Geometry check sheet. Reference: the model listing, model coordinates, mm. Face numbers are marked on the shaded views. A direction names the side the tool comes from. Coordinates: 2 decimals unless noted, no trailing zeros. Loops run counter-clockwise (first coordinate to the right, second up) from the corner with the lowest first, then second, coordinate; pieces in that order, holes last. Notation, with made-up numbers: (-29.75, -26.75) - (11.25, -26.75) arc R31 ccw to (11.25, 8.25) - close; hole circle Ø8 at (23, 89). An arc over 180 degrees is marked (long way). Write item = value, one per line. Start each with the question number.
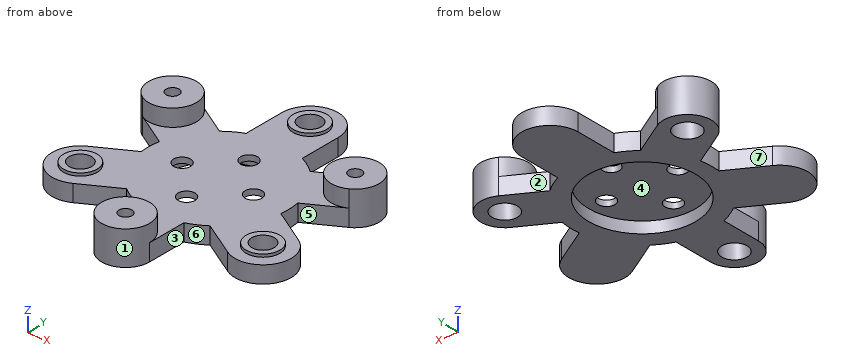
Autodesk Inventor part; units mm, degrees
ref_plane "YZ Plane" through (0, 0, 0) normal (1, 0, 0) x (0, 1, 0)
ref_plane "XZ Plane" through (0, 0, 0) normal (0, 1, 0) x (-1, 0, 0)
ref_plane "XY Plane" through (0, 0, 0) normal (0, 0, 1) x (1, 0, 0)
sketch "Skizze1" plane through (0, 0, 0) normal (0, 0, 1) x (1, 0, 0)
  circle A0 centre (0, 0) radius 18.75 construction
  circle A1 centre (0, 0) radius 9.5
  circle A2 centre (0, 18.75) radius 2
  line L0 (0, 0) -> (-16.238, -9.375) construction
  line L1 (0, 33.1) -> (0, -32.35) construction
  line L2 (-32.2953, 0) -> (32.2953, 0) construction
  circle A3 centre (0, 0) radius 6.35 construction
  circle A4 centre (0, 6.35) radius 1.5
  circle A5 centre (0, -6.35) radius 1.5
  circle A6 centre (6.35, 0) radius 1.5
  circle A7 centre (-6.35, 0) radius 1.5
  arc A8 (-5, 11.4564) -> (5, 11.4564) centre (0, 0) ccw
  arc A9 (5, 18.75) -> (-5, 18.75) centre (0, 18.75) ccw
  line L3 (-5, 18.75) -> (-5, 11.4564)
  line L4 (5, 18.75) -> (5, 11.4564)
  circle A10 centre (16.238, -9.375) radius 2
  arc A11 (13.738, -13.7051) -> (18.738, -5.0449) centre (16.238, -9.375) ccw
  line L5 (18.738, -5.0449) -> (12.4216, -1.3981)
  line L6 (13.738, -13.7051) -> (7.4216, -10.0583)
  circle A12 centre (-16.238, -9.375) radius 2
  arc A13 (-18.738, -5.0449) -> (-13.738, -13.7051) centre (-16.238, -9.375) ccw
  line L7 (-18.738, -5.0449) -> (-12.4216, -1.3981)
  line L8 (-13.738, -13.7051) -> (-7.4216, -10.0583)
  circle A14 centre (0, 18.75) radius 3
  circle A15 centre (16.238, -9.375) radius 3
  circle A16 centre (-16.238, -9.375) radius 3
  circle A17 centre (0, -18.75) radius 1.15
  circle A18 centre (16.238, 9.375) radius 1.15
  circle A19 centre (-16.238, 9.375) radius 1.15
  circle A20 centre (16.238, 9.375) radius 2.25
  circle A21 centre (0, -18.75) radius 2.25
  circle A22 centre (-16.238, 9.375) radius 2.25
  arc A23 (18.363, 5.6944) -> (14.113, 13.0556) centre (16.238, 9.375) ccw
  arc A24 (-4.25, -18.75) -> (4.25, -18.75) centre (0, -18.75) ccw
  arc A25 (-14.113, 13.0556) -> (-18.363, 5.6944) centre (-16.238, 9.375) ccw
  line L9 (18.363, 5.6944) -> (12.3054, 2.1971)
  line L10 (14.113, 13.0556) -> (8.0554, 9.5583)
  line L11 (4.25, -11.7553) -> (4.25, -18.75)
  line L12 (-4.25, -11.7553) -> (-4.25, -18.75)
  line L13 (-8.0554, 9.5583) -> (-14.113, 13.0556)
  line L14 (-12.3054, 2.1971) -> (-18.363, 5.6944)
  circle A26 centre (0, -18.75) radius 4.25
  circle A27 centre (16.238, 9.375) radius 4.25
  circle A28 centre (-16.238, 9.375) radius 4.25
  dimension "d0" = 37.5
  dimension "d1" = 4
  dimension "d2" = 30
  dimension "d3" = 19
  dimension "d4" = 12.7
  dimension "d5" = 3
  dimension "d7" = 3
  dimension "d8" = 3
  dimension "d17" = 1
  dimension "d20" = 2.3
  dimension "d22" = 2
  dimension "d23" = 4.5
extrude "Extrusion1" add sketch "Skizze1" along normal blind 3 contours A1 | A2 | L3 A9 L4 A8 | A8 L14 A28 L13 | A28 A25 | A8 L8 A13 L7 | L10 A27 L9 A8 | A8 L11 A26 L12 | A23 A27 | A26 A24 | L5 A11 L6 A8 | A10 | A12 | A14 | A15 | A16
extrude "Extrusion3" cut sketch "Skizze1" along normal blind 2 contours A1
extrude "Extrusion4" cut sketch "Skizze1" against normal blind 2 from surface at 3 contours A2 | A10 | A12
extrude "Extrusion5" add sketch "Skizze1" along normal blind 0.5 from surface at 3 contours A14 | A15 | A16
extrude "Extrusion6" add sketch "Skizze1" along normal blind 3 from surface at 3 contours A28 A25 | A23 A27 | A26 A24 | A20 | A21 | A22
properties part number "PlanetaryHolderTop"
(1) Draft check along X on the marked faces 5, 6 and 7. Enter one of: pulls with the +X half, pulls with the -X half, needs draft (parallel to the pull), parting line crosses it, or undercut.
(2) Depth check by flat-ended pin: pin 1 (3.5 mm diameter, centred on x = 0, y = -18.75, fed in from -Z); pin 2 (6.5 mm diameter, centred on x = -1, y = 20, fed in from +Z); pin 3 (3 mm diameter, centred on y = 7.5, z = 2.5, fed in from +X). Enter the tip coordinate at first touch or a pass-through.
(3) Sectioned sample at B-B on z = 5.35. Enter the section's corners in (x, y) (3 decimals), plus the area to 3 significant figures.
(4) Scan lines: line 1 (Y direction, x = 0, z = 2.7); line 2 (Z direction, x = 3.5, y = 7); line 3 (Y direction, x = 17.5, z = 2.7). Record each from-to range of solid material in increasing order.
(5) Sectioned sample at C-C on x = 0. Count the separate pieces of the cut face and the enclosed holes in it, plus the area to 4 significant figures.
(6) Tool access check on the marked faces 1, 2, 3 and 4. Record the directions out of +Z, -Z, +X, -X, +Y, -Y that give a thin tool (end or side, any length) a straight path to the whole face; none if there is none.
(7) Sectioned sample at A-A on y = 0. Enter the section's corners in (x, z).
(8) Sectioned sample at D-D on x = 6.35. Enter the section's corners in (y, z).
Working result:
q1.face_5 = pulls with the +X half
q1.face_6 = undercut
q1.face_7 = pulls with the -X half
q2.pin_1 = 3
q2.pin_2 = 3.5
q2.pin_3 = 20.47
q3.outline = (-18.363, 5.694) arc R4.25 ccw to (-14.113, 13.056) arc R4.25 ccw to start; circle Ø8.5 at (0, -18.75); circle Ø8.5 at (16.238, 9.375); hole circle Ø2.3 at (-16.238, 9.375); hole circle Ø2.3 at (0, -18.75); hole circle Ø2.3 at (16.238, 9.375)
q3.area = 158 mm2
q4.line_1 = -23 to -21, -16.5 to -7.85, -4.85 to 4.85, 7.85 to 16.75, 20.75 to 23.75
q4.line_2 = 2 to 3
q4.line_3 = -14.21 to -10.93, -7.82 to -4.33, 5.2 to 7.51, 11.24 to 13.43
q5.separate_pieces = 4
q5.enclosed_holes = 0
q5.area = 94.35 mm2
q6.face_1 = +Z
q6.face_2 = +Z, -Z, +Y
q6.face_3 = +Z, -Z, -Y
q6.face_4 = -Z
q7.outline = (-12.5, 0) - (-9.5, 0) - (-9.5, 2) - (-7.85, 2) - (-7.85, 3) - (-12.5, 3) - close; (-4.85, 2) - (4.85, 2) - (4.85, 3) - (-4.85, 3) - close; (7.85, 2) - (9.5, 2) - (9.5, 0) - (12.5, 0) - (12.5, 3) - (7.85, 3) - close
q8.outline = (-10.77, 0) - (-7.07, 0) - (-7.07, 2) - (-1.5, 2) - (-1.5, 3) - (-10.77, 3) - close; (1.5, 2) - (7.07, 2) - (7.07, 0) - (10.77, 0) - (10.77, 3) - (1.5, 3) - close
